```python
from build123d import *

# Parameters (mm, degrees)
F0_W     = 76.2
F0_H     = 76.2
F1_DEPTH = 76.2
F2_R     = 39.306587
F3_DEPTH = 101.6


with BuildPart() as f1:
    # F0 (on Front) → F1 (new body)
    with BuildSketch(Plane.XZ):
        with Locations((-46.311049, 48.602506)):
            Rectangle(F0_W, F0_H)
    extrude(amount=F1_DEPTH)

    # F2 (on face) → F3 (cut)
    with BuildSketch(Plane.XZ.offset(76.2)):
        with BuildLine():
            ThreePointArc((-8.211049, 41.7134), (10.932512, 56.060384), (18.212613, 78.848802))
            ThreePointArc((18.212613, 78.848802), (-17.147175, 117.956736), (-59.60796, 86.702506))
            Line((-59.60796, 86.702506), (-8.211049, 86.702506))
            Line((-8.211049, 86.702506), (-8.211049, 41.7134))
        make_face()
        with Locations((-21.093974, 78.848802)):
            Circle(F2_R)
    extrude(amount=-F3_DEPTH, mode=Mode.SUBTRACT)


solid = f1.part
```
Input: part model. Units: mm. Frame: model coordinates. Coordinates: 2 decimals unless noted, no trailing zeros. Write each loop counter-clockwise with the first axis right and the second up, starting at its lowest first coordinate (ties: lowest second). Pieces come first, ordered by that corner, then holes. Notation, with made-up numbers: (-19, -37) -> (17, -37) arc R26 cw to (17, -16) -> close; hole circle Ø2 at (87, 24). An arc over 180 degrees is marked (long way). Write each question's results on one line, items separated by ' | '.
Item 1: Pin query (flat end, axial travel): pin 1 Ø1 at (y, z) = (-50, 61.5) entering from +X; pin 2 Ø3 at (x, y) = (-26, -11) entering from +Z; pin 3 Ø5 at (y, z) = (-10, 54.5) entering from +X. Return the tip coordinate at first contact, or that it passes through.
Conclusion:
pin 1: stops at x = -56.11 | pin 2: stops at z = 40.07 | pin 3: stops at x = -49.8
Item 2: Mould query, pull axis X, two halves, no side actions, for faces 1 (the cylindrical face through (-47.42, -38.63, 49.66)), 2 (the flat face through (-8.211, -38, 26)), 3 (the flat face through (-84.411, -38, 48)). Classes: +X half, -X half, draft (parallel to the pull), parting line (faces both ways), or undercut.
Conclusion:
face 1: undercut | face 2: +X half | face 3: -X half
Item 3: Section query A-A on y = -69.5. Return loops of the section in (x, z).
Conclusion:
outline: (-84.41, 10.5) -> (-8.21, 10.5) -> (-8.21, 41.71) arc R39.31 cw to (-59.61, 86.7) -> (-84.41, 86.7) -> close
Item 4: Material intervals for probe 1 along Z at (x, y) = (-20.5, -14); probe 2 along Z at (x, y) = (-20, -9); probe 3 along X at (y, z) = (-60.5, 79.5), sorted ascending.
Conclusion:
probe 1: z = 10.5 to 39.55 | probe 2: z = 10.5 to 39.56 | probe 3: x = -84.41 to -60.4
Item 5: Section query C-C on z = 64. Return loops of the section in (x, y).
Conclusion:
outline: (-84.41, -76.2) -> (-57.49, -76.2) -> (-57.49, 0) -> (-84.41, 0) -> close
Item 6: Section query B-B on x = -58.5. Return loops of the section in (y, z).
Conclusion:
outline: (-76.2, 10.5) -> (0, 10.5) -> (0, 66.77) -> (-76.2, 66.77) -> close
